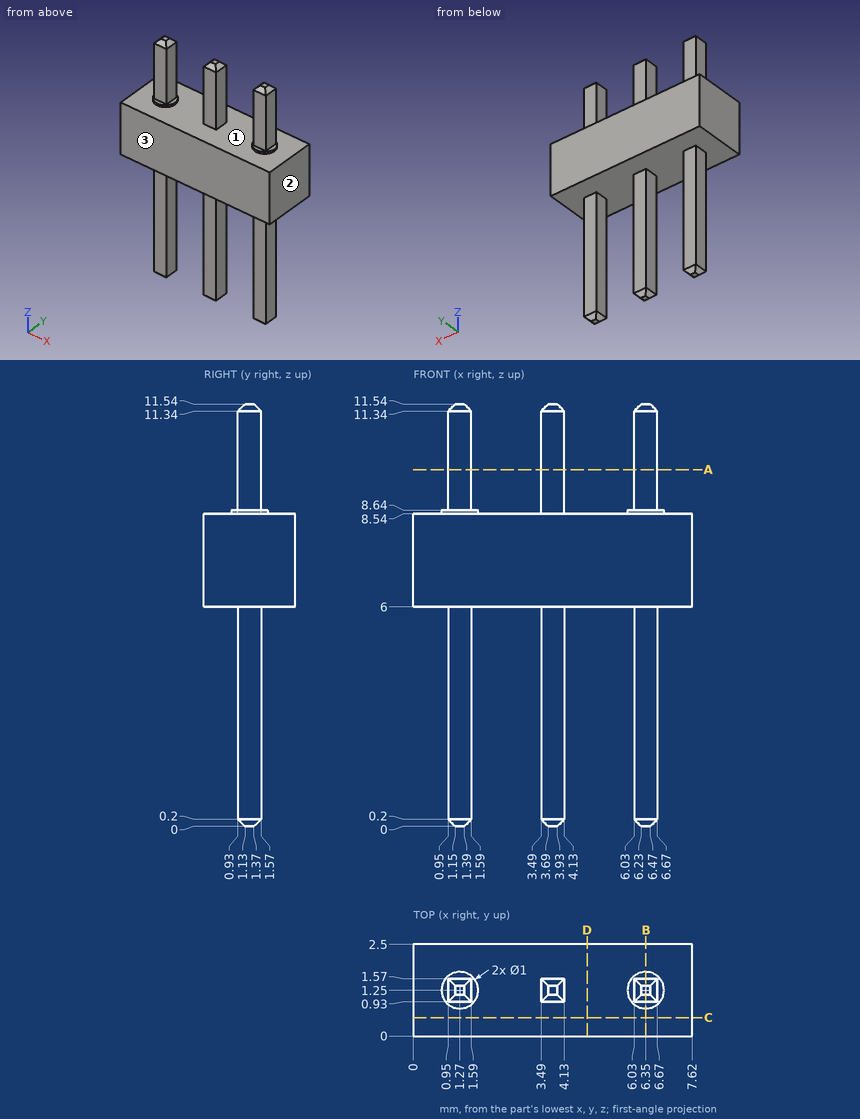
Geometry check sheet. Reference: drawing and pictorial views, mm from the part's lowest x, y, z. Give positions to 0.01 mm unless a question says otherwise; leave off trailing zeros. Write each loop counter-clockwise with the first axis right and the second up, starting at its lowest first coordinate (ties: lowest second). Pieces come first, ordered by that corner, then holes. Notation, with made-up numbers: (-18, -16.75) -> (20, -16.75) arc R32 cw to (20, 16.25) -> close; hole circle Ø4 at (67, 6.25). An arc over 180 degrees is marked (long way). One line per item, written item: value. Start each with the question number.
Item 1: Material ranges on probe 1 along X at (y, z) = (1.5, 11); probe 2 along Z at (x, y) = (3.75, 0.6); probe 3 along Y at (x, z) = (6.5, 3.75), recorded low to high. Write a range as from..to.
Item 2: Section check C-C on y = 0.5. Record the cut outline in (x, z).
Item 3: Section check A-A on z = 9.75. Record the cut outline in (x, y).
Item 4: Gauge pin test, flat ends, axial feed: pin 1 (0.7 mm diameter, centred on x = 6.5, z = 3.5, fed in from -Y); pin 2 (1.2 mm diameter, centred on x = 2, y = 1, fed in from +Z); pin 3 (0.7 mm diameter, centred on y = 1, z = 1.5, fed in from -X). Record the tip position at first contact, or that the pin passes through.
Item 5: Section check B-B on x = 6.35. Record the cut outline in (y, z), then the cut area to 3 significant figures.
Item 6: Section check D-D on x = 4.75. Record the cut outline in (y, z), then the cut area to 3 significant figures.
Item 7: Draft check along X on the marked faces 1, 2 and 3. Enter one of: +X half, -X half, draft (parallel to the pull), parting line (faces both ways), or undercut.
Results list:
1. probe 1: 0.95..1.59, 3.49..4.13, 6.03..6.67
1. probe 2: 6..8.54
1. probe 3: 0.93..1.57
2. outline: (0, 6) -> (7.62, 6) -> (7.62, 8.54) -> (0, 8.54) -> close
3. outline: (0.95, 0.93) -> (1.59, 0.93) -> (1.59, 1.57) -> (0.95, 1.57) -> close; (3.49, 0.93) -> (4.13, 0.93) -> (4.13, 1.57) -> (3.49, 1.57) -> close; (6.03, 0.93) -> (6.67, 0.93) -> (6.67, 1.57) -> (6.03, 1.57) -> close
4. pin 1: y = 0.93
4. pin 2: z = 11.52
4. pin 3: x = 0.95
5. outline: (0, 6) -> (0.93, 6) -> (0.93, 0.2) -> (1.13, 0) -> (1.37, 0) -> (1.57, 0.2) -> (1.57, 6) -> (2.5, 6) -> (2.5, 8.54) -> (1.75, 8.54) -> (1.75, 8.64) -> (1.57, 8.64) -> (1.57, 11.34) -> (1.37, 11.54) -> (1.13, 11.54) -> (0.93, 11.34) -> (0.93, 8.64) -> (0.75, 8.64) -> (0.75, 8.54) -> (0, 8.54) -> close
5. area: 12.1 mm²
6. outline: (0, 6) -> (2.5, 6) -> (2.5, 8.54) -> (0, 8.54) -> close
6. area: 6.35 mm²
7. face 1: undercut
7. face 2: +X half
7. face 3: draft
